from build123d import *

# Parameters (mm, degrees)
SKETCH1_W           = 17.2
SKETCH1_H           = 6
SKETCH1_W_2         = 13.2
SKETCH1_H_2         = 2
BOSS_EXTRUDE1_DEPTH = 13
CUT_EXTRUDE1_DEPTH  = 13
SKETCH4_W           = 17.2
SKETCH4_H           = 1.968955047
BOSS_EXTRUDE2_DEPTH = 7
SKETCH5_R           = 1.6
CUT_EXTRUDE2_DEPTH  = 4
CUT_EXTRUDE3_START  = -7
SKETCH6_W           = 11.206506984
SKETCH6_H           = 2.48590404
CUT_EXTRUDE3_DEPTH  = 7
CUT_EXTRUDE4_START  = -17.2
CUT_EXTRUDE4_DEPTH  = 17.2
FILLET1_R           = 8


with BuildPart() as part:
    # Sketch1 → Boss-Extrude1 (new body)
    with BuildSketch(Plane(origin=(0, 0, 0), x_dir=(1, 0, 0), z_dir=(0, 1, 0))):
        with Locations((6.6, 1)):
            Rectangle(SKETCH1_W, SKETCH1_H)
        with Locations((6.6, 1)):
            Rectangle(SKETCH1_W_2, SKETCH1_H_2, mode=Mode.SUBTRACT)
    extrude(amount=BOSS_EXTRUDE1_DEPTH)

    # Sketch2 → Cut-Extrude1 (cut)
    with BuildSketch(Plane.XY.offset(2)):
        with BuildLine():
            Line((2, 5.2), (11.2, 5.2))
            ThreePointArc((11.2, 5.2), (11.907106781, 4.907106781), (12.2, 4.2))
            Line((12.2, 4.2), (12.2, 3))
            ThreePointArc((12.2, 3), (11.907106781, 2.292893219), (11.2, 2))
            Line((11.2, 2), (2, 2))
            ThreePointArc((2, 2), (1.292893219, 2.292893219), (1, 3))
            Line((1, 3), (1, 4.2))
            ThreePointArc((1, 4.2), (1.292893219, 4.907106781), (2, 5.2))
        make_face()
    extrude(amount=-CUT_EXTRUDE1_DEPTH, mode=Mode.SUBTRACT)

    # Sketch4 → Boss-Extrude2 (add)
    with BuildSketch(Plane(origin=(0, 0, -4), x_dir=(-1, 0, 0), z_dir=(0, 0, -1))):
        with Locations((-6.6, 0.984477524)):
            Rectangle(SKETCH4_W, SKETCH4_H)
    extrude(amount=BOSS_EXTRUDE2_DEPTH)

    # Sketch5 → Cut-Extrude2 (cut)
    with BuildSketch(Plane(origin=(0, 1.968955047, 0), x_dir=(1, 0, 0), z_dir=(0, 1, 0))):
        with Locations(Location((6.6, 7.5, 0), (0, 0, 270))):
            Circle(SKETCH5_R)
    extrude(amount=-CUT_EXTRUDE2_DEPTH, mode=Mode.SUBTRACT)

    # Sketch6 → Cut-Extrude3 (cut)
    with BuildSketch(Plane(origin=(0, 0, -11), x_dir=(-1, 0, 0), z_dir=(0, 0, -1)).offset(CUT_EXTRUDE3_START)):
        with Locations((-6.603253492, 1.995400835)):
            Rectangle(SKETCH6_W, SKETCH6_H)
    extrude(amount=CUT_EXTRUDE3_DEPTH, mode=Mode.SUBTRACT)

    # Sketch7 → Cut-Extrude4 (cut)
    with BuildSketch(Plane(origin=(15.2, 0, 0), x_dir=(0, 0, -1), z_dir=(1, 0, 0)).offset(CUT_EXTRUDE4_START)):
        Polygon((0, 13), (-2, 6.017150325), (-2, 13), align=None)
    extrude(amount=CUT_EXTRUDE4_DEPTH, mode=Mode.SUBTRACT)

    # Fillet1
    # the kernel refuses this fillet: 8 mm, written as the material it takes off along each edge
    with BuildSketch(Plane(origin=(-4.807712941, 6.017150325, 2), x_dir=(0, -1, 0), z_dir=(1, 0, 0))) as fillet1_piece_1:
        with BuildLine():
            CenterArc((FILLET1_R * 0.140385647075, FILLET1_R), FILLET1_R, 254.01743912, 15.98256088)
            Line((-FILLET1_R * 0.134959116702, FILLET1_R * 0.0386544528314), (0, 0))
            Line((0, 0), (FILLET1_R * 0.140385647075, 0))
        make_face()
    extrude(amount=22.815425883, mode=Mode.SUBTRACT)


solid = part.part
The listing builds one solid part. Answer for the finished solid, in the listing's coordinates (mm). A direction names the side the tool comes from. Coordinates: 2 decimals unless noted, no trailing zeros. Write each loop counter-clockwise with the first axis right and the second up, starting at its lowest first coordinate (ties: lowest second). Pieces come first, ordered by that corner, then holes. Notation, with made-up numbers: (47.25, 46) - (58.25, 46) arc R19 ccw to (58.25, 61) - close; hole circle Ø1 at (16.5, 87.5). An arc over 180 degrees is marked (long way). Return JSON: item names as keys, results as strings.
1. The part is cut by section B-B on z = -3. Determine the outline of the cut face in (x, y), then the cut area to 3 significant figures.
Final values:
{"outline": "(-2, 0) - (15.2, 0) - (15.2, 13) - (-2, 13) - close; hole (1, 3) arc R1 ccw to (2, 2) - (11.2, 2) arc R1 ccw to (12.2, 3) - (12.2, 4.2) arc R1 ccw to (11.2, 5.2) - (2, 5.2) arc R1 ccw to (1, 4.2) - close", "area": "189 mm^2"}
2. Each of these flat-tipped pins is pushed along its axis until it touches: pin 1 Ø6 at (x, y) = (3.5, 10) entering from +Z; pin 2 Ø7.5 at (x, z) = (6, -9) entering from +Y; pin 3 Ø3.5 at (x, z) = (13.5, -7.5) entering from +Y. Where does it stop, or does it pass through?
Final values:
{"pin 1": "z = 1.72", "pin 2": "y = 0.75", "pin 3": "y = 1.97"}
3. Consider line 1 along X through (y, z) = (6.5, -1.5); line 2 along Y through (x, z) = (7, -2.5); line 3 along X through (y, z) = (0.35, -7.5). Determine where each line is inside the solid, lowest interval first.
Final values:
{"line 1": "-2 to 0, 13.2 to 15.2", "line 2": "0 to 2, 5.2 to 13", "line 3": "-2 to 5, 8.2 to 15.2"}
4. Which of the six approach directions +Z, -Z, +X, -X, +Y, -Y give full straight-line access (tool end or side, diameter ignored) to faces 1 (the face through (0, 6, -1)), 2 (the face through (12.207, 1, -7)), 3 (the face through (6, 1, 2)), 4 (the face through (1.301, 2.285, 1.014))?
Final values:
{"face 1": "+Y, -Y", "face 2": "-Z, +Y", "face 3": "+Z, +X, -X, +Y, -Y", "face 4": "+Z, -Z"}
5. For a pull along Z with two mould halves and no side action, classify faces 5 (the face through (6.7, 0.6, -11)), 6 (the face through (6.48, 10.09, 0.834)), 7 (the face through (7, 8, 0)), 8 (the face through (6.5, 13, -2.5)) as +Z half, -Z half, draft (parallel to the pull), parting line (faces both ways), or undercut.
Final values:
{"face 5": "-Z half", "face 6": "+Z half", "face 7": "undercut", "face 8": "draft"}
6. The part is cut by section A-A on x = 6.6. Determine the outline of the cut face in (y, z).
Final values:
{"outline": "(0, -11) - (0.75, -11) - (0.75, -9.1) - (0, -9.1) - close; (0, -5.9) - (0.75, -5.9) - (0.75, -4) - (2, -4) - (2, -2) - (0, -2) - close; (0, 0) - (2, 0) - (2, 2) - (0, 2) - close; (5.2, -4) - (13, -4) - (13, -2) - (5.2, -2) - close; (5.2, 0) - (13, 0) - (7.1, 1.69) arc R8 ccw to (5.2, 1.99) - close"}
7. The part is cut by section D-D on y = 6.5. Determine the outline of the cut face in (x, z).
Final values:
{"outline": "(-2, -4) - (15.2, -4) - (15.2, 1.84) - (-2, 1.84) - close; hole (0, -2) - (13.2, -2) - (13.2, 0) - (0, 0) - close"}
8. The part is cut by section C-C on z = -8. Determine the outline of the cut face in (x, y).
Final values:
{"outline": "(-2, 0) - (5.08, 0) - (5.08, 0.75) - (1, 0.75) - (1, 1.97) - (-2, 1.97) - close; (8.12, 0) - (15.2, 0) - (15.2, 1.97) - (12.21, 1.97) - (12.21, 0.75) - (8.12, 0.75) - close"}
